Input: part model. Units: mm. Frame: model coordinates. A direction names the side the tool comes from. Coordinates: 2 decimals unless noted, no trailing zeros. Order: outer loops, then holes, each group sorted by start corner. A loop starts at its lowest first (then second) coordinate and runs counter-clockwise, first axis right, second up.
from build123d import *

# Parameters (mm, degrees)
F1_DEPTH  = 38
F4_DEPTH  = 13
F5_DEPTH  = 26
F6_R      = 19
F7_DEPTH  = 26.001
F8_R      = 28.5
F9_DEPTH  = 1
F10_R     = 19
F11_DEPTH = 26.001
F12_R     = 28.5
F13_DEPTH = 1
F14_R     = 6


with BuildPart() as f1:
    # F0 (on Front) → F1 (new body, symmetric)
    with BuildSketch(Plane.XZ):
        Polygon((0, 139), (0, 0), (127, 0), (127, 50), (38, 139), align=None)
    extrude(amount=F1_DEPTH, both=True)

    # F3 (on Front) → F4 (cut, symmetric)
    with BuildSketch(Plane.XZ):
        Polygon((127, 50), (38, 139), (12, 139), (127, 24), align=None)
    extrude(amount=F4_DEPTH, both=True, mode=Mode.SUBTRACT)

    # F2 (on face) → F5 (join)
    with BuildSketch(Plane(origin=(0, 0, 0), x_dir=(1, 0, 0), z_dir=(0, 0, -1))):
        with BuildLine():
            ThreePointArc((0, -89), (38, -127), (76, -89))
            Line((76, -89), (76, 89))
            ThreePointArc((76, 89), (38, 127), (0, 89))
            Line((0, 89), (0, -89))
        make_face()
    extrude(amount=-F5_DEPTH)

    # F6 (on face) → F7 (cut, through all)
    with BuildSketch(Plane.XY.offset(26)):
        with Locations((38, -89)):
            Circle(F6_R)
    extrude(amount=-F7_DEPTH, mode=Mode.SUBTRACT)

    # F8 (on face) → F9 (cut)
    with BuildSketch(Plane.XY.offset(26)):
        with Locations((38, -89)):
            Circle(F8_R)
    extrude(amount=-F9_DEPTH, mode=Mode.SUBTRACT)

    # F10 (on face) → F11 (cut, through all)
    with BuildSketch(Plane.XY.offset(26)):
        with Locations((38, 89)):
            Circle(F10_R)
    extrude(amount=-F11_DEPTH, mode=Mode.SUBTRACT)

    # F12 (on face) → F13 (cut)
    with BuildSketch(Plane.XY.offset(26)):
        with Locations((38, 89)):
            Circle(F12_R)
    extrude(amount=-F13_DEPTH, mode=Mode.SUBTRACT)

    # F14
    f14_edges = [f1.edges().sort_by_distance(p)[0] for p in [
        (76, -63.5, 26),
        (76, 63.5, 26),
        (0, 63.5, 26),
        (0, -63.5, 26),
        (38, -127, 26),
        (38, 127, 26),
    ]]
    fillet(f14_edges, radius=F14_R)


solid = f1.part
Item 1: Cut plane C-C on y = -81.5. Return loops of the section in (x, z), then the cut area to 3 significant figures.
Response values:
outline: (0, 0) - (20.54, 0) - (20.54, 25) - (10.5, 25) - (10.5, 26) - (6, 26) arc R6 ccw to (0, 20) - close; (55.46, 0) - (76, 0) - (76, 20) arc R6 ccw to (70, 26) - (65.5, 26) - (65.5, 25) - (55.46, 25) - close
area: 1,030 mm2
Item 2: Cut plane D-D on y = 47. Return loops of the section in (x, z).
Response values:
outline: (0, 0) - (76, 0) - (76, 20) arc R6 ccw to (70, 26) - (6, 26) arc R6 ccw to (0, 20) - close
Item 3: Access query for faces 1 (the face through (31.82, 61.18, 25.51)), 2 (the face through (69, 0, 82)), 3 (the face through (76, 64, 10)), 4 (the face through (74.289, 63.143, 24.196)), 5 (the face through (23, -62, 26)). Directions: +Z, -Z, +X, -X, +Y, -Y. A direction counts if a zero-diameter tool reaches every point of the face in a straight line with its end or side. Return the directions, or none.
Response values:
face 1: +Z
face 2: +Z, +X
face 3: +Z, -Z, +X, +Y
face 4: +Z, +X, +Y
face 5: +Z, +X, -X, -Y
Item 4: Cut plane A-A on z = 87. Return loops of the section in (x, y).
Response values:
outline: (0, -38) - (90, -38) - (90, -13) - (64, -13) - (64, 13) - (90, 13) - (90, 38) - (0, 38) - close
Item 5: Pin query (flat end, axial travel): pin 1 Ø6 at (y, z) = (85, 20) entering from +X; pin 2 Ø23 at (x, y) = (38, -89) entering from -Z; pin 3 Ø8 at (x, z) = (43, 44) entering from +Y; pin 4 Ø5 at (x, z) = (31.5, 17.5) entering from -Y. Return the tip coordinate at first contact, or that it passes through.
Response values:
pin 1: stops at x = 76
pin 2: passes through
pin 3: stops at y = 38
pin 4: stops at y = -126.79
Item 6: Ray query, probe 1 along Y at (x, z) = (38, 10.75); probe 2 along Y at (x, z) = (8.5, 47); probe 3 along Z at (x, y) = (9, -44). Return the intervals inside material, ascending.
Response values:
probe 1: y = -127 to -108, -70 to 70, 108 to 127
probe 2: y = -38 to 38
probe 3: z = 0 to 26
Item 7: Cut plane B-B on x = 116.5. Return loops of the section in (y, z).
Response values:
outline: (-38, 0) - (38, 0) - (38, 60.5) - (13, 60.5) - (13, 34.5) - (-13, 34.5) - (-13, 60.5) - (-38, 60.5) - close
Item 8: Draft query along X for faces 6 (the face through (38, 60, 26)), 7 (the face through (35.53, 107.84, 12.68)), 8 (the face through (83, -26, 94)). Return one class per face: pulls with the +X half, pulls with the -X half, needs draft (parallel to the pull), parting line crosses it, or undercut.
Response values:
face 6: needs draft
face 7: undercut
face 8: pulls with the +X half
